```python
from build123d import *

# Parameters (mm, degrees)
F0_W           = 19
F0_H           = 19
F1_DEPTH       = 9.5
F3_DEPTH       = 19.001
F5_DEPTH       = 3
F6_R           = 2
F8_DEPTH       = 12.501
F9_R           = 2
F10_R          = 2.99999
F11_R          = 2
F13_ANGLE_BACK = 50
F13_ANGLE      = 100


# Not quite as in the source:
# - a fillet or chamfer is up to 0.001 mm smaller than in the source, because OpenCascade refuses the exact size


with BuildPart() as f1:
    # F0 (on Front) → F1 (new body, symmetric)
    with BuildSketch(Plane.XZ):
        with Locations((9.5, 9.5)):
            Rectangle(F0_W, F0_H)
    extrude(amount=F1_DEPTH, both=True)

    # F2 (on face) → F3 (cut, through all)
    with BuildSketch(Plane.XZ.offset(9.5)):
        with BuildLine():
            ThreePointArc((6, 19), (9.8076118446, 9.8076118446), (19, 6))
            Line((19, 6), (19, 19))
            Line((19, 19), (6, 19))
        make_face()
    extrude(amount=-F3_DEPTH, mode=Mode.SUBTRACT)

    # F4 (on Front) → F5 (join, symmetric)
    with BuildSketch(Plane.XZ):
        Polygon((0, 18), (0, 0), (18, 0), (18, 11.5), (24.5, 11.5), (24.5, 24.5), (11.5, 24.5), (11.5, 18), align=None)
    extrude(amount=F5_DEPTH, both=True)

    # F6
    f6_edges = [f1.edges().sort_by_distance(p)[0] for p in [
        (0, 0, 0),
    ]]
    fillet(f6_edges, radius=F6_R)

    # F7 (on face) → F8 (cut, through all)
    with BuildSketch(Plane.XZ.offset(3)):
        Polygon((17.5, 24.5), (24.5, 17.5), (24.5, 24.5), align=None)
    extrude(amount=-F8_DEPTH, mode=Mode.SUBTRACT)

    # F9
    f9_edges = [f1.edges().sort_by_distance(p)[0] for p in [
        (0, -9.5, 10.5),
        (0, 9.5, 10.5),
        (0, 0, 19),
        (3, 9.5, 19),
        (3, -9.5, 19),
        (19, 9.5, 3),
        (19, 0, 0),
        (19, -9.5, 3),
    ]]
    fillet(f9_edges, radius=F9_R)

    # F10 (radius 3 in the source; OpenCascade refuses exactly that, so slightly less here)
    f10_edges = [f1.edges().sort_by_distance(p)[0] for p in [
        (14.5, -3, 24.5),
        (21, -3, 21),
        (24.5, -3, 14.5),
        (14.5, 3, 24.5),
        (21, 3, 21),
        (24.5, 3, 14.5),
    ]]
    fillet(f10_edges, radius=F10_R)

    # F11
    f11_edges = [f1.edges().sort_by_distance(p)[0] for p in [
        (17.118519, 2.162797, 23.579023),
        (23.579023, 2.162797, 17.118519),
    ]]
    fillet(f11_edges, radius=F11_R)

    # F12 (on Front) → F13 (revolve)
    with BuildSketch(Plane.XZ, mode=Mode.PRIVATE) as f13_sk:
        with BuildLine():
            Line((14.434, 20.434), (11.434, 20.434))
            ThreePointArc((11.434, 20.434), (14.0700389693, 14.0700389693), (20.434, 11.434))
            Line((20.434, 11.434), (20.434, 14.434))
            ThreePointArc((20.434, 14.434), (16.1913593129, 16.1913593129), (14.434, 20.434))
        make_face()
    revolve(f13_sk.sketch.rotate(Axis((20.434, 0, 20.434), (0.7071067812, 0, -0.7071067812)), -F13_ANGLE_BACK), axis=Axis((20.434, 0, 20.434), (0.7071067812, 0, -0.7071067812)), revolution_arc=F13_ANGLE)


solid = f1.part
```
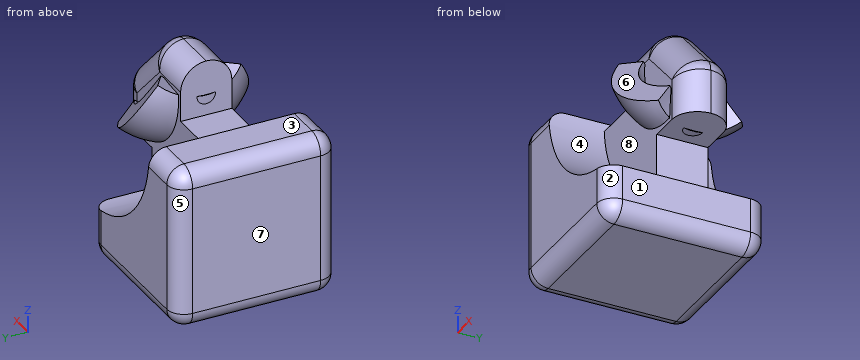
Design review of the part built by this model. Coordinates are the model's own, in mm. Face numbers are marked on the shaded views. A direction names the side the tool comes from. Coordinates: 2 decimals unless noted, no trailing zeros. Write each loop counter-clockwise with the first axis right and the second up, starting at its lowest first coordinate (ties: lowest second). Pieces come first, ordered by that corner, then holes.
1) Add section D-D (x = 10.5). Write out the cut boundary in (y, z).
2) Add section A-A (z = 5). Write out the cut boundary in (x, y).
3) Add section C-C (z = 11). Write out the cut boundary in (x, y).
4) Machinability: for the marked faces 1, 2, 3, 4 and 5, which of the approach directions +Z, -Z, +X, -X, +Y, -Y give a long, thin tool a straight path to every point of the face, cutting with its end or side? Answer none if there is none.
5) Mouldability with a two-part tool opening along X and no side actions: class the marked faces 6, 7 and 8 as +X half, -X half, draft (parallel to the pull), parting line (faces both ways), or undercut.
6) Add section B-B (x = 4.75). Write out the cut boundary in (y, z).
7) To check wall thickness, follow L1, parallel to X at y = 4.25, z = 5.5; L2, parallel to X at y = -2, z = 8.5. State the ranges of each line that lie inside material, in increasing order.
8) Insertion check: pin 1 (3 mm diameter, centred on y = 3.5, z = 19.5, fed in from -X); pin 2 (2.5 mm diameter, centred on x = 8.5, y = 1, fed in from +Z); pin 3 (3 mm diameter, centred on y = 2.5, z = 3, fed in from +X). Each pin has a flat end and moves straight along its axis. Give the tip position at first contact, or say it passes through.
Check result:
1. outline: (-9.5, 2) arc R2 ccw to (-7.5, 0) - (7.5, 0) arc R2 ccw to (9.5, 2) - (9.5, 9.16) - (3, 9.16) - (3, 18) - (-3, 18) - (-3, 9.16) - (-9.5, 9.16) - close
2. outline: (0, -7.5) arc R2 ccw to (2, -9.5) - (17, -9.5) arc R2 ccw to (19, -7.5) - (19, 7.5) arc R2 ccw to (17, 9.5) - (2, 9.5) arc R2 ccw to (0, 7.5) - close
3. outline: (0, -7.5) arc R2 ccw to (2, -9.5) - (8.75, -9.5) - (8.75, -3) - (18, -3) - (18, 3) - (8.75, 3) - (8.75, 9.5) - (2, 9.5) arc R2 ccw to (0, 7.5) - close
4. face 1: -Z, +X, +Y, -Y
4. face 2: +Z, -Z, +X, -Y
4. face 3: +Z, -X, +Y, -Y
4. face 4: none
4. face 5: +Z, -Z, -X, +Y
5. face 6: +X half
5. face 7: -X half
5. face 8: undercut
6. outline: (-9.5, 2) arc R2 ccw to (-7.5, 0) - (7.5, 0) arc R2 ccw to (9.5, 2) - (9.5, 17) arc R2 ccw to (7.5, 19) - (-7.5, 19) arc R2 ccw to (-9.5, 17) - close
7. L1: x = 0 to 19
7. L2: x = 0 to 18
8. pin 1: stops at x = 0.27
8. pin 2: stops at z = 18
8. pin 3: stops at x = 19
